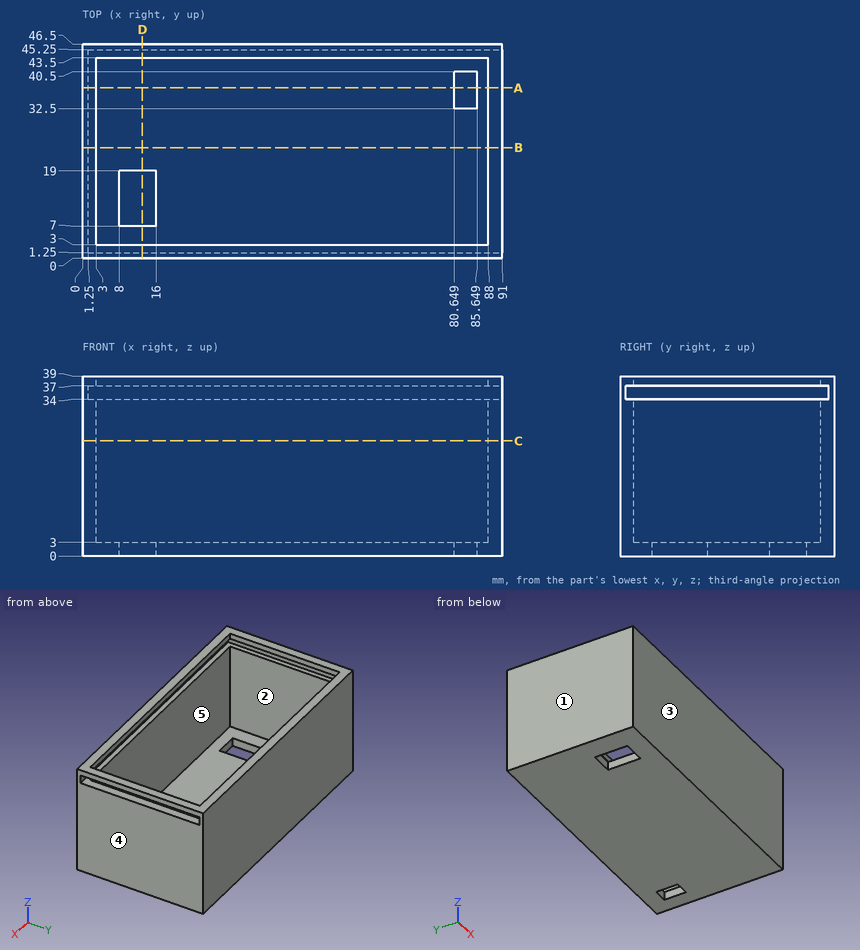
Job drawing, mm, ordinate dimensions from the low corner. One solid piece. A direction names the side the tool comes from. Give positions to 0.01 mm unless a question says otherwise; leave off trailing zeros. Loops run counter-clockwise (first coordinate to the right, second up) from the corner with the lowest first, then second, coordinate; pieces in that order, holes last. Notation, with made-up numbers: (-30, 63) -> (-8, 63) arc R15 cw to (-8, 87) -> close; hole circle Ø2 at (47, 71). An arc over 180 degrees is marked (long way). Use a Markdown table: item, result. Add a question column.
(1) Slice it at B-B on y = 24. List the corners of the cut face in (x, z).
(2) Wall check: line 1 along Y through (x, z) = (65.5, 16); line 2 along X through (y, z) = (20, 30.5); line 3 along Y through (x, z) = (51, 34.5). Give the ranges that are in metal, low to high.
(3) Drop a flat-ended pin along its axis: pin 1 Ø1.5 at (x, y) = (42, 41.5) entering from +Z. Give the stop position or say it passes through.
(4) Slice it at D-D on x = 13. List the corners of the cut face in (y, z), and give its area (3 significant figures).
(5) Slice it at C-C on z = 25. List the corners of the cut face in (x, y), and give its area (3 significant figures).
(6) Slice it at A-A on y = 37. List the corners of the cut face in (x, z), and give its area (3 significant figures).
(7) Mould opens along X. For the marked faces 3, 4 and 5 say: +X half, -X half, draft (parallel to the pull), parting line (faces both ways), or undercut.
(8) Tool access for the marked faces 1 and 2: list every direction of +Z, -Z, +X, -X, +Y, -Y with a clear straight run to the whole face (end or side of a thin tool).
Filled sheet:
| question | item | result |
|---|---|---|
| 1 | outline | (0, 0) -> (91, 0) -> (91, 34) -> (88, 34) -> (88, 3) -> (3, 3) -> (3, 34) -> (1.25, 34) -> (1.25, 37) -> (3, 37) -> (3, 39) -> (0, 39) -> close; (88, 37) -> (91, 37) -> (91, 39) -> (88, 39) -> close |
| 2 | line 1 | 0 to 3, 43.5 to 46.5 |
| 2 | line 2 | 0 to 3, 88 to 91 |
| 2 | line 3 | 0 to 1.25, 45.25 to 46.5 |
| 3 | pin 1 | z = 3 |
| 4 | outline | (0, 0) -> (7, 0) -> (7, 3) -> (3, 3) -> (3, 34) -> (1.25, 34) -> (1.25, 37) -> (3, 37) -> (3, 39) -> (0, 39) -> close; (19, 0) -> (46.5, 0) -> (46.5, 39) -> (43.5, 39) -> (43.5, 37) -> (45.25, 37) -> (45.25, 34) -> (43.5, 34) -> (43.5, 3) -> (19, 3) -> close |
| 4 | area | 309 mm2 |
| 5 | outline | (0, 0) -> (91, 0) -> (91, 46.5) -> (0, 46.5) -> close; hole (3, 3) -> (88, 3) -> (88, 43.5) -> (3, 43.5) -> close |
| 5 | area | 789 mm2 |
| 6 | outline | (0, 0) -> (80.65, 0) -> (80.65, 3) -> (3, 3) -> (3, 34) -> (1.25, 34) -> (1.25, 37) -> (3, 37) -> (3, 39) -> (0, 39) -> close; (85.65, 0) -> (91, 0) -> (91, 34) -> (88, 34) -> (88, 3) -> (85.65, 3) -> close; (88, 37) -> (91, 37) -> (91, 39) -> (88, 39) -> close |
| 6 | area | 460 mm2 |
| 7 | face 3 | draft |
| 7 | face 4 | +X half |
| 7 | face 5 | undercut |
| 8 | face 1 | +Z, -Z, -X, +Y, -Y |
| 8 | face 2 | +Z |
